Read the model definition and answer for the solid it produces. Units are mm, in the model's axes. A direction names the side the tool comes from. Round coordinates to 2 decimals unless told otherwise and drop trailing zeros. Order: outer loops, then holes, each group sorted by start corner. A loop starts at its lowest first (then second) coordinate and runs counter-clockwise, first axis right, second up. Notation, with made-up numbers: (60, 13) - (84, 13) arc R29 cw to (84, 44) - close; hole circle Ø5 at (-11.75, -26.5). An arc over 180 degrees is marked (long way). Put each result on its own line as item: value. Start each with the question number.
Q1. Section C-C on z = -16 is taken. Give the vertices of the cut face in (x, y).
Q2. Section D-D on y = 95 is taken. Give the vertices of the cut face in (x, z), then the cut area to 3 significant figures.
Q3. Each of these flat-tipped pins is pushed along its axis until it touches: pin 1 Ø6.5 at (x, y) = (35, 28) entering from +Z; pin 2 Ø5 at (x, y) = (-21, -14) entering from -Z. Where does it stop, or does it pass through?
Q4. Section B-B on x = -35 is taken. Give the vertices of the cut face in (y, z), then the cut area to 3 significant figures.
Q5. For a pull along Y with two mould halves and no side action, classify faces 1 (the face through (-1, 31, 0)), 2 (the face through (-21, 26, -2)) as pulls with the +Y half, pulls with the -Y half, needs draft (parallel to the pull), parting line crosses it, or undercut.
Q6. Which of the six approach directions +Z, -Z, +X, -X, +Y, -Y give full straight-line access (tool end or side, diameter ignored) to faces 3 (the face through (47, 29, -27)), 4 (the face through (-7, -30, -2))?
Q7. Section A-A on y = 14 is taken. State how many separate pieces and enclosed holes the cut face has, then the cut area to 3 significant figures.
Q8. Find the intervals of material crossed by line 1 along Y through (x, z) = (-7, -2); line 2 along X through (y, z) = (-13.5, -28.5); line 3 along Y through (x, z) = (30.5, -40), in increasing order. Write a range as from..to.
from build123d import *

# Parameters (mm, degrees)
F0_W     = 104
F0_H     = 150
F0_R     = 2
F1_DEPTH = 50
F2_T     = -5
F3_DEPTH = 25


# Not quite as in the source:
# - a feature names something its author has since deleted; it is built from what else it names


with BuildPart() as f1:
    # F0 (on Top) → F1 (new body)
    with BuildSketch(Plane.XY):
        with Locations((0, 30)):
            Rectangle(F0_W, F0_H)
        with Locations((-35, -28)):
            Circle(F0_R, mode=Mode.SUBTRACT)
        with Locations((-35, -14)):
            Circle(F0_R, mode=Mode.SUBTRACT)
        with Locations((-21, -28)):
            Circle(F0_R, mode=Mode.SUBTRACT)
        with Locations((-7, -28)):
            Circle(F0_R, mode=Mode.SUBTRACT)
        with Locations((-21, -14)):
            Circle(F0_R, mode=Mode.SUBTRACT)
        with Locations((-7, -14)):
            Circle(F0_R, mode=Mode.SUBTRACT)
        with Locations((-35, 0)):
            Circle(F0_R, mode=Mode.SUBTRACT)
        with Locations((-35, 14)):
            Circle(F0_R, mode=Mode.SUBTRACT)
        with Locations((-35, 28)):
            Circle(F0_R, mode=Mode.SUBTRACT)
        with Locations((-21, 0)):
            Circle(F0_R, mode=Mode.SUBTRACT)
        with Locations((-7, 0)):
            Circle(F0_R, mode=Mode.SUBTRACT)
        with Locations((-21, 14)):
            Circle(F0_R, mode=Mode.SUBTRACT)
        with Locations((-21, 28)):
            Circle(F0_R, mode=Mode.SUBTRACT)
        with Locations((-7, 14)):
            Circle(F0_R, mode=Mode.SUBTRACT)
        with Locations((-7, 28)):
            Circle(F0_R, mode=Mode.SUBTRACT)
        with Locations((7, -28)):
            Circle(F0_R, mode=Mode.SUBTRACT)
        with Locations((21, -28)):
            Circle(F0_R, mode=Mode.SUBTRACT)
        with Locations((7, -14)):
            Circle(F0_R, mode=Mode.SUBTRACT)
        with Locations((21, -14)):
            Circle(F0_R, mode=Mode.SUBTRACT)
        with Locations((35, -28)):
            Circle(F0_R, mode=Mode.SUBTRACT)
        with Locations((35, -14)):
            Circle(F0_R, mode=Mode.SUBTRACT)
        with Locations((7, 0)):
            Circle(F0_R, mode=Mode.SUBTRACT)
        with Locations((21, 0)):
            Circle(F0_R, mode=Mode.SUBTRACT)
        with Locations((7, 14)):
            Circle(F0_R, mode=Mode.SUBTRACT)
        with Locations((7, 28)):
            Circle(F0_R, mode=Mode.SUBTRACT)
        with Locations((21, 14)):
            Circle(F0_R, mode=Mode.SUBTRACT)
        with Locations((21, 28)):
            Circle(F0_R, mode=Mode.SUBTRACT)
        with Locations((35, 0)):
            Circle(F0_R, mode=Mode.SUBTRACT)
        with Locations((35, 14)):
            Circle(F0_R, mode=Mode.SUBTRACT)
        with Locations((35, 28)):
            Circle(F0_R, mode=Mode.SUBTRACT)
        with Locations((7, -28)):
            Circle(F0_R)
        with Locations((35, 14)):
            Circle(F0_R)
        with Locations((21, 0)):
            Circle(F0_R)
        with Locations((21, 28)):
            Circle(F0_R)
        with Locations((7, 28)):
            Circle(F0_R)
        with Locations((35, -28)):
            Circle(F0_R)
        with Locations((-7, -14)):
            Circle(F0_R)
        with Locations((-7, -28)):
            Circle(F0_R)
        with Locations((7, 14)):
            Circle(F0_R)
        with Locations((-35, 28)):
            Circle(F0_R)
        with Locations((-35, 14)):
            Circle(F0_R)
        with Locations((-35, 0)):
            Circle(F0_R)
        with Locations((-35, -14)):
            Circle(F0_R)
        with Locations((-35, -28)):
            Circle(F0_R)
        with Locations((-21, 28)):
            Circle(F0_R)
        with Locations((-21, 14)):
            Circle(F0_R)
        with Locations((-21, 0)):
            Circle(F0_R)
        with Locations((-21, -14)):
            Circle(F0_R)
        with Locations((-21, -28)):
            Circle(F0_R)
        with Locations((-7, 28)):
            Circle(F0_R)
        with Locations((-7, 14)):
            Circle(F0_R)
        with Locations((-7, 0)):
            Circle(F0_R)
        with Locations((35, 0)):
            Circle(F0_R)
        with Locations((21, -14)):
            Circle(F0_R)
        with Locations((21, 14)):
            Circle(F0_R)
        with Locations((7, 0)):
            Circle(F0_R)
        with Locations((35, -14)):
            Circle(F0_R)
        with Locations((21, -28)):
            Circle(F0_R)
        with Locations((7, -14)):
            Circle(F0_R)
        with Locations((35, 28)):
            Circle(F0_R)
    extrude(amount=-F1_DEPTH)

    # F2
    f2_openings = [f1.faces().sort_by_distance(p)[0] for p in [
        (0, 30, -50),
    ]]
    offset(amount=F2_T, openings=f2_openings)

    # F0 (on Top) → F3 (cut)
    with BuildSketch(Plane.XY):
        with Locations((7, -14)):
            Circle(F0_R)
        with Locations((35, -14)):
            Circle(F0_R)
        with Locations((21, -28)):
            Circle(F0_R)
        with Locations((7, 0)):
            Circle(F0_R)
        with Locations((21, 14)):
            Circle(F0_R)
        with Locations((21, -14)):
            Circle(F0_R)
        with Locations((35, 0)):
            Circle(F0_R)
        with Locations((-7, 0)):
            Circle(F0_R)
        with Locations((-7, 14)):
            Circle(F0_R)
        with Locations((-7, 28)):
            Circle(F0_R)
        with Locations((-21, -28)):
            Circle(F0_R)
        with Locations((-21, -14)):
            Circle(F0_R)
        with Locations((-21, 0)):
            Circle(F0_R)
        with Locations((-21, 14)):
            Circle(F0_R)
        with Locations((-35, -28)):
            Circle(F0_R)
        with Locations((-35, -14)):
            Circle(F0_R)
        with Locations((-35, 0)):
            Circle(F0_R)
        with Locations((7, 14)):
            Circle(F0_R)
        with Locations((-7, -28)):
            Circle(F0_R)
        with Locations((-7, -14)):
            Circle(F0_R)
        with Locations((7, 28)):
            Circle(F0_R)
        with Locations((35, -28)):
            Circle(F0_R)
        with Locations((21, 28)):
            Circle(F0_R)
        with Locations((21, 0)):
            Circle(F0_R)
        with Locations((35, 14)):
            Circle(F0_R)
        with Locations((7, -28)):
            Circle(F0_R)
        with Locations((35, 28)):
            Circle(F0_R)
        with Locations((-21, 28)):
            Circle(F0_R)
        with Locations((-35, 14)):
            Circle(F0_R)
        with Locations((-35, 28)):
            Circle(F0_R)
    extrude(amount=-F3_DEPTH, mode=Mode.SUBTRACT)


solid = f1.part
Findings:
1. outline: (-52, -45) - (52, -45) - (52, 105) - (-52, 105) - close; hole (-47, -40) - (47, -40) - (47, 100) - (-47, 100) - close
2. outline: (-52, -50) - (-47, -50) - (-47, -5) - (47, -5) - (47, -50) - (52, -50) - (52, 0) - (-52, 0) - close
2. area: 970 mm2
3. pin 1: z = 0
3. pin 2: z = -5
4. outline: (-45, -50) - (-40, -50) - (-40, -5) - (-30, -5) - (-30, 0) - (-45, 0) - close; (-26, -5) - (-16, -5) - (-16, 0) - (-26, 0) - close; (-12, -5) - (-2, -5) - (-2, 0) - (-12, 0) - close; (2, -5) - (12, -5) - (12, 0) - (2, 0) - close; (16, -5) - (26, -5) - (26, 0) - (16, 0) - close; (30, -5) - (100, -5) - (100, -50) - (105, -50) - (105, 0) - (30, 0) - close
4. area: 1,100 mm2
5. face 1: needs draft
5. face 2: undercut
6. face 3: -Z
6. face 4: +Z, -Z
7. separate pieces: 7
7. enclosed holes: 0
7. area: 850 mm2
8. line 1: -45..-30, -26..-16, -12..-2, 2..12, 16..26, 30..105
8. line 2: -52..-47, 47..52
8. line 3: -45..-40, 100..105
